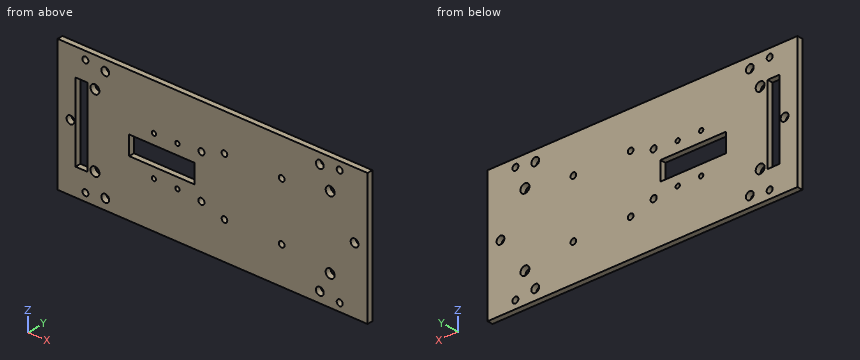
```python
from build123d import *

# Parameters (mm, degrees)
SKETCH1_W           = 165.1
SKETCH1_H           = 69.85
BOSS_EXTRUDE1_DEPTH = 3
CUT_EXTRUDE1_REACH  = 91.684
SKETCH6_R           = 1.5
SKETCH6_R_2         = 1.625
SKETCH6_W           = 34.925
SKETCH6_H           = 10
CUT_EXTRUDE3_REACH  = 91.684
SKETCH8_R           = 2.38125
SKETCH9_R           = 2.0828
CUT_EXTRUDE5_DEPTH  = 5.08
SKETCH10_R          = 2.0828
CUT_EXTRUDE6_DEPTH  = 5.08
SKETCH11_R          = 1.125
SKETCH11_R_2        = 1.125000036
CUT_EXTRUDE7_DEPTH  = 41.91
SKETCH13_R          = 1.5875
CUT_EXTRUDE9_DEPTH  = 5
SKETCH15_W          = 6.35
SKETCH15_H          = 41.275
CUT_EXTRUDE10_DEPTH = 7.62


with BuildPart() as part:
    # Sketch1 → Boss-Extrude1 (new body)
    with BuildSketch(Plane(origin=(0, 0, 0), x_dir=(1, 0, 0), z_dir=(0, 1, 0))):
        Rectangle(SKETCH1_W, SKETCH1_H)
    extrude(amount=BOSS_EXTRUDE1_DEPTH)

    # Sketch6 → Cut-Extrude1 (cut, up to next)
    with BuildSketch(Plane.XZ, mode=Mode.PRIVATE) as cut_extrude1_sk1:
        with Locations(Location((6.35, 15.25, 0), (0, 0, 270))):
            Circle(SKETCH6_R)
    cut_extrude1_tool1 = extrude(cut_extrude1_sk1.sketch, amount=-CUT_EXTRUDE1_REACH, mode=Mode.PRIVATE) & part.part
    # Sketch6 → Cut-Extrude1 (cut, up to next)
    with BuildSketch(Plane.XZ, mode=Mode.PRIVATE) as cut_extrude1_sk2:
        with Locations(Location((36.85, 15.25, 0), (0, 0, 270))):
            Circle(SKETCH6_R)
    cut_extrude1_tool2 = extrude(cut_extrude1_sk2.sketch, amount=-CUT_EXTRUDE1_REACH, mode=Mode.PRIVATE) & part.part
    # Sketch6 → Cut-Extrude1 (cut, up to next)
    with BuildSketch(Plane.XZ, mode=Mode.PRIVATE) as cut_extrude1_sk3:
        with Locations(Location((6.35, -15.25, 0), (0, 0, 270))):
            Circle(SKETCH6_R)
    cut_extrude1_tool3 = extrude(cut_extrude1_sk3.sketch, amount=-CUT_EXTRUDE1_REACH, mode=Mode.PRIVATE) & part.part
    # Sketch6 → Cut-Extrude1 (cut, up to next)
    with BuildSketch(Plane.XZ, mode=Mode.PRIVATE) as cut_extrude1_sk4:
        with Locations(Location((36.85, -15.25, 0), (0, 0, 270))):
            Circle(SKETCH6_R)
    cut_extrude1_tool4 = extrude(cut_extrude1_sk4.sketch, amount=-CUT_EXTRUDE1_REACH, mode=Mode.PRIVATE) & part.part
    # Sketch6 → Cut-Extrude1 (cut, up to next)
    with BuildSketch(Plane.XZ, mode=Mode.PRIVATE) as cut_extrude1_sk5:
        with Locations(Location((-5.924999961, 11.500993, 0), (0, 0, 270))):
            Circle(SKETCH6_R_2)
    cut_extrude1_tool5 = extrude(cut_extrude1_sk5.sketch, amount=-CUT_EXTRUDE1_REACH, mode=Mode.PRIVATE) & part.part
    # Sketch6 → Cut-Extrude1 (cut, up to next)
    with BuildSketch(Plane.XZ, mode=Mode.PRIVATE) as cut_extrude1_sk6:
        with Locations(Location((-5.924999961, -11.500993, 0), (0, 0, 270))):
            Circle(SKETCH6_R_2)
    cut_extrude1_tool6 = extrude(cut_extrude1_sk6.sketch, amount=-CUT_EXTRUDE1_REACH, mode=Mode.PRIVATE) & part.part
    # Sketch6 → Cut-Extrude1 (cut, up to next)
    with BuildSketch(Plane.XZ, mode=Mode.PRIVATE) as cut_extrude1_sk7:
        with Locations((-26.9875, 0)):
            Rectangle(SKETCH6_W, SKETCH6_H)
    cut_extrude1_tool7 = extrude(cut_extrude1_sk7.sketch, amount=-CUT_EXTRUDE1_REACH, mode=Mode.PRIVATE) & part.part
    add(cut_extrude1_tool1.solids().sort_by_distance((6.35, 0, 15.25))[0], mode=Mode.SUBTRACT)
    add(cut_extrude1_tool2.solids().sort_by_distance((36.85, 0, 15.25))[0], mode=Mode.SUBTRACT)
    add(cut_extrude1_tool3.solids().sort_by_distance((6.35, 0, -15.25))[0], mode=Mode.SUBTRACT)
    add(cut_extrude1_tool4.solids().sort_by_distance((36.85, 0, -15.25))[0], mode=Mode.SUBTRACT)
    add(cut_extrude1_tool5.solids().sort_by_distance((-5.925, 0, 11.500993))[0], mode=Mode.SUBTRACT)
    add(cut_extrude1_tool6.solids().sort_by_distance((-5.925, 0, -11.500993))[0], mode=Mode.SUBTRACT)
    add(cut_extrude1_tool7.solids().sort_by_distance((-26.9875, 0, 0))[0], mode=Mode.SUBTRACT)

    # Sketch8 → Cut-Extrude3 (cut, up to next)
    with BuildSketch(Plane(origin=(0, 3, 0), x_dir=(1, 0, 0), z_dir=(0, 1, 0)), mode=Mode.PRIVATE) as cut_extrude3_sk1:
        with Locations(Location((-62.6618, -19.05, 0), (0, 0, 270))):
            Circle(SKETCH8_R)
    cut_extrude3_tool1 = extrude(cut_extrude3_sk1.sketch, amount=-CUT_EXTRUDE3_REACH, mode=Mode.PRIVATE) & part.part
    # Sketch8 → Cut-Extrude3 (cut, up to next)
    with BuildSketch(Plane(origin=(0, 3, 0), x_dir=(1, 0, 0), z_dir=(0, 1, 0)), mode=Mode.PRIVATE) as cut_extrude3_sk2:
        with Locations(Location((-62.6618, 19.05, 0), (0, 0, 270))):
            Circle(SKETCH8_R)
    cut_extrude3_tool2 = extrude(cut_extrude3_sk2.sketch, amount=-CUT_EXTRUDE3_REACH, mode=Mode.PRIVATE) & part.part
    # Sketch8 → Cut-Extrude3 (cut, up to next)
    with BuildSketch(Plane(origin=(0, 3, 0), x_dir=(1, 0, 0), z_dir=(0, 1, 0)), mode=Mode.PRIVATE) as cut_extrude3_sk3:
        with Locations(Location((62.6618, 19.05, 0), (0, 0, 270))):
            Circle(SKETCH8_R)
    cut_extrude3_tool3 = extrude(cut_extrude3_sk3.sketch, amount=-CUT_EXTRUDE3_REACH, mode=Mode.PRIVATE) & part.part
    # Sketch8 → Cut-Extrude3 (cut, up to next)
    with BuildSketch(Plane(origin=(0, 3, 0), x_dir=(1, 0, 0), z_dir=(0, 1, 0)), mode=Mode.PRIVATE) as cut_extrude3_sk4:
        with Locations(Location((62.6618, -19.05, 0), (0, 0, 270))):
            Circle(SKETCH8_R)
    cut_extrude3_tool4 = extrude(cut_extrude3_sk4.sketch, amount=-CUT_EXTRUDE3_REACH, mode=Mode.PRIVATE) & part.part
    add(cut_extrude3_tool1.solids().sort_by_distance((-62.6618, 3, 19.05))[0], mode=Mode.SUBTRACT)
    add(cut_extrude3_tool2.solids().sort_by_distance((-62.6618, 3, -19.05))[0], mode=Mode.SUBTRACT)
    add(cut_extrude3_tool3.solids().sort_by_distance((62.6618, 3, -19.05))[0], mode=Mode.SUBTRACT)
    add(cut_extrude3_tool4.solids().sort_by_distance((62.6618, 3, 19.05))[0], mode=Mode.SUBTRACT)

    # Sketch9 → Cut-Extrude5 (cut)
    with BuildSketch(Plane(origin=(0, 3, 0), x_dir=(1, 0, 0), z_dir=(0, 1, 0))):
        with Locations(Location((-75.692, 0, 0), (0, 0, 270))):
            Circle(SKETCH9_R)
        with Locations(Location((75.692, 0, 0), (0, 0, 270))):
            Circle(SKETCH9_R)
    extrude(amount=-CUT_EXTRUDE5_DEPTH, mode=Mode.SUBTRACT)

    # Sketch10 → Cut-Extrude6 (cut)
    with BuildSketch(Plane(origin=(0, 3, 0), x_dir=(1, 0, 0), z_dir=(0, 1, 0))):
        with Locations(Location((57.15, -29.337, 0), (0, 0, 270))):
            Circle(SKETCH10_R)
        with Locations(Location((57.15, 29.337, 0), (0, 0, 270))):
            Circle(SKETCH10_R)
        with Locations(Location((-57.15, -29.337, 0), (0, 0, 270))):
            Circle(SKETCH10_R)
        with Locations(Location((-57.15, 29.337, 0), (0, 0, 270))):
            Circle(SKETCH10_R)
    extrude(amount=-CUT_EXTRUDE6_DEPTH, mode=Mode.SUBTRACT)

    # Sketch11 → Cut-Extrude7 (cut)
    with BuildSketch(Plane(origin=(0, 3, 0), x_dir=(1, 0, 0), z_dir=(0, 1, 0))):
        with Locations(Location((-31.2375, 10.5, 0), (0, 0, 270))):
            Circle(SKETCH11_R)
        with Locations(Location((-18.7375, 10.5, 0), (0, 0, 270))):
            Circle(SKETCH11_R_2)
        with Locations(Location((-18.7375, -10.5, 0), (0, 0, 270))):
            Circle(SKETCH11_R_2)
        with Locations(Location((-31.2375, -10.5, 0), (0, 0, 270))):
            Circle(SKETCH11_R_2)
    extrude(amount=-CUT_EXTRUDE7_DEPTH, mode=Mode.SUBTRACT)

    # Sketch13 → Cut-Extrude9 (cut)
    with BuildSketch(Plane.XZ):
        with Locations(Location((-67.742170098, 30.689580734, 0), (0, 0, 270))):
            Circle(SKETCH13_R)
        with Locations(Location((67.742170098, 30.689580734, 0), (0, 0, 270))):
            Circle(SKETCH13_R)
        with Locations(Location((67.742170098, -30.689580734, 0), (0, 0, 270))):
            Circle(SKETCH13_R)
        with Locations(Location((-67.742170098, -30.689580734, 0), (0, 0, 270))):
            Circle(SKETCH13_R)
    extrude(amount=-CUT_EXTRUDE9_DEPTH, mode=Mode.SUBTRACT)

    # Sketch15 → Cut-Extrude10 (cut)
    with BuildSketch(Plane.XZ):
        with Locations((-69.85, 0)):
            Rectangle(SKETCH15_W, SKETCH15_H)
    extrude(amount=-CUT_EXTRUDE10_DEPTH, mode=Mode.SUBTRACT)


solid = part.part
```
Part model, mm, in its own coordinate system. Coordinates: 2 decimals unless noted, no trailing zeros. Order: outer loops, then holes, each group sorted by start corner. A loop starts at its lowest first (then second) coordinate and runs counter-clockwise, first axis right, second up. Notation, with made-up numbers: (61.25, -0.5) -> (78.25, -0.5) arc R19 cw to (78.25, 13.5) -> close; hole circle Ø8 at (30.5, 1.5). An arc over 180 degrees is marked (long way). Put each result on its own line as item: value. Start each with the question number.
(1) Probe line 1 along X through (y, z) = (0.8, 4) (3 decimals); line 2 along Z through (x, y) = (-5.5, 2.45) (3 decimals); line 3 along X through (y, z) = (2.5, 7.5) (3 decimals). List the from-to ranges inside material, lowest first. Write a range as [from, to].
(2) Band-saw the part on C-C (x = -12.5). Give the cut face in (y, z) (3 decimals), then the cut area to 3 significant figures.
(3) Band-saw the part on D-D (z = 0). Give the cut face in (x, y) (3 decimals).
(4) Pin check, flat tip, straight feed: pin 1 Ø1 at (x, z) = (54.5, -20) entering from -Y. Stop position of the tip, or through.
(5) Band-saw the part on B-B (x = 57.15). Give the cut face in (y, z) (3 decimals), then the cut area to 3 significant figures.
(6) Band-saw the part on A-A (z = 19.05). Give the cut face in (x, y) (3 decimals), then the cut area to 3 significant figures.
Determined:
1. line 1: x = [-82.55, -73.025], [-66.675, -44.45], [-9.525, 82.55]
1. line 2: z = [-34.925, -13.069], [-9.933, 9.933], [13.069, 34.925]
1. line 3: x = [-82.55, -73.025], [-66.675, 82.55]
2. outline: (0, -34.925) -> (3, -34.925) -> (3, -5) -> (0, -5) -> close; (0, 5) -> (3, 5) -> (3, 34.925) -> (0, 34.925) -> close
2. area: 180 mm²
3. outline: (-82.55, 0) -> (-77.775, 0) -> (-77.775, 3) -> (-82.55, 3) -> close; (-73.609, 0) -> (-73.025, 0) -> (-73.025, 3) -> (-73.609, 3) -> close; (-66.675, 0) -> (-44.45, 0) -> (-44.45, 3) -> (-66.675, 3) -> close; (-9.525, 0) -> (73.609, 0) -> (73.609, 3) -> (-9.525, 3) -> close; (77.775, 0) -> (82.55, 0) -> (82.55, 3) -> (77.775, 3) -> close
4. pin 1: stops at y = 0
5. outline: (0, -34.925) -> (3, -34.925) -> (3, -31.42) -> (0, -31.42) -> close; (0, -27.254) -> (3, -27.254) -> (3, 27.254) -> (0, 27.254) -> close; (0, 31.42) -> (3, 31.42) -> (3, 34.925) -> (0, 34.925) -> close
5. area: 185 mm²
6. outline: (-82.55, 0) -> (-73.025, 0) -> (-73.025, 3) -> (-82.55, 3) -> close; (-66.675, 0) -> (-65.043, 0) -> (-65.043, 3) -> (-66.675, 3) -> close; (-60.281, 0) -> (60.281, 0) -> (60.281, 3) -> (-60.281, 3) -> close; (65.043, 0) -> (82.55, 0) -> (82.55, 3) -> (65.043, 3) -> close
6. area: 448 mm²
